CAD build for the part. Positions are in the model's coordinates, mm. A direction names the side the tool comes from. Give positions to 0.01 mm unless a question says otherwise; leave off trailing zeros. Write each loop counter-clockwise with the first axis right and the second up, starting at its lowest first coordinate (ties: lowest second). Pieces come first, ordered by that corner, then holes. Notation, with made-up numbers: (54.25, 42.5) -> (103.25, 42.5) arc R22 ccw to (103.25, 60.5) -> close; hole circle Ø1 at (89, 14). An arc over 180 degrees is marked (long way). Answer in a Markdown table with one row per item. Add a question column.
```python
from build123d import *

# Parameters (mm, degrees)
F0_W     = 88.9
F0_H     = 38.1
F1_DEPTH = 50.8
F2_W     = 63.5
F2_H     = 19.05
F3_DEPTH = 50.801
F4_R     = 6.35
F5_DEPTH = 19.051
F6_R     = 6.35
F7_DEPTH = 19.051


with BuildPart() as f1:
    # F0 (on Front) → F1 (new body)
    with BuildSketch(Plane.XZ):
        Rectangle(F0_W, F0_H)
    extrude(amount=F1_DEPTH)

    # F2 (on face) → F3 (cut, through all)
    with BuildSketch(Plane.XZ.offset(50.8)):
        with Locations((0, 9.525)):
            Rectangle(F2_W, F2_H)
    extrude(amount=-F3_DEPTH, mode=Mode.SUBTRACT)

    # F4 (on face) → F5 (cut, through all)
    with BuildSketch(Plane.XY):
        with Locations((-19.05, -38.1)):
            Circle(F4_R)
    extrude(amount=-F5_DEPTH, mode=Mode.SUBTRACT)

    # F6 (on face) → F7 (cut, through all)
    with BuildSketch(Plane.XY):
        with Locations((6.35, -12.7)):
            Circle(F6_R)
    extrude(amount=-F7_DEPTH, mode=Mode.SUBTRACT)


solid = f1.part
```
Item 1: Slice it at B-B, the plane y = -38.1. List the corners of the cut face in (x, z).
Item 2: Slice it at A-A, the plane x = 6.35. List the corners of the cut face in (y, z), then the cut area to 3 significant figures.
Item 3: Which spindle directions (+Z, -Z, +X, -X, +Y, -Y) get a long thin tool onto all of the face, cutting with end or side? Do faces 1 (the face through (44.45, -25, 0)), 2 (the face through (-31.75, -26, 9)). Say none if no direction does.
Item 4: Slice it at D-D, the plane y = -29. List the corners of the cut face in (x, z).
Item 5: Slice it at C-C, the plane z = 6. List the corners of the cut face in (x, y), then the cut area to 3 significant figures.
Item 6: Probe L1, parallel to X at y = -14, z = 12.5; L2, parallel to X at y = -38, z = -3; L3, parallel to Y at x = 6, z = -14. List the from-to ranges inside material, lowest first. Write a range as from..to.
Item 7: Mould opens along Y. For faces 3 (the face through (-1, -25, -19.05)), 4 (the face through (-1, 0, -8)), 5 (the face through (-25.394, -37.821, -9.392)), 6 (the face through (-1, -50.8, -8)) say: released by +Y, released by -Y, zero draft, split by the parting line, or undercut.
Item 8: Drop a flat-ended pin along its axis: pin 1 Ø2 at (x, y) = (7.5, -23) entering from +Z. Give the stop position or say it passes through.
Answer key:
| question | item | result |
|---|---|---|
| 1 | outline | (-44.45, -19.05) -> (-25.4, -19.05) -> (-25.4, 0) -> (-31.75, 0) -> (-31.75, 19.05) -> (-44.45, 19.05) -> close; (-12.7, -19.05) -> (44.45, -19.05) -> (44.45, 19.05) -> (31.75, 19.05) -> (31.75, 0) -> (-12.7, 0) -> close |
| 2 | outline | (-50.8, -19.05) -> (-19.05, -19.05) -> (-19.05, 0) -> (-50.8, 0) -> close; (-6.35, -19.05) -> (0, -19.05) -> (0, 0) -> (-6.35, 0) -> close |
| 2 | area | 726 mm² |
| 3 | face 1 | +Z, -Z, +X, +Y, -Y |
| 3 | face 2 | +Z, +Y, -Y |
| 4 | outline | (-44.45, -19.05) -> (44.45, -19.05) -> (44.45, 19.05) -> (31.75, 19.05) -> (31.75, 0) -> (-31.75, 0) -> (-31.75, 19.05) -> (-44.45, 19.05) -> close |
| 5 | outline | (-44.45, -50.8) -> (-31.75, -50.8) -> (-31.75, 0) -> (-44.45, 0) -> close; (31.75, -50.8) -> (44.45, -50.8) -> (44.45, 0) -> (31.75, 0) -> close |
| 5 | area | 1,290 mm² |
| 6 | L1 | x = -44.45..-31.75, 31.75..44.45 |
| 6 | L2 | x = -44.45..-25.4, -12.7..44.45 |
| 6 | L3 | y = -50.8..-19.04, -6.36..0 |
| 7 | face 3 | zero draft |
| 7 | face 4 | released by +Y |
| 7 | face 5 | undercut |
| 7 | face 6 | released by -Y |
| 8 | pin 1 | stops at z = 0 |
